```python
from build123d import *

# Parameters (mm, degrees)
F0_R     = 2
F0_R_2   = 4.5
F0_R_3   = 5.5
F1_DEPTH = 10
F0_R_4   = 3
F2_DEPTH = 4
F3_R     = 4
F3_R_2   = 2
F4_DEPTH = 5


with BuildPart() as f1:
    # F0 (on Front) → F1 (new body)
    with BuildSketch(Plane.XZ):
        with BuildLine():
            Line((20, -40), (10, 0))
            ThreePointArc((10, 0), (0, 10), (-10, 0))
            Line((-10, 0), (-20, -40))
            ThreePointArc((-20, -40), (0, -60), (20, -40))
        make_face()
        with Locations((-12.5, -40)):
            Circle(F0_R, mode=Mode.SUBTRACT)
        with Locations((0, -49.5)):
            Circle(F0_R, mode=Mode.SUBTRACT)
        with Locations((0, -40)):
            Circle(F0_R_2, mode=Mode.SUBTRACT)
        with Locations((0, -30.5)):
            Circle(F0_R, mode=Mode.SUBTRACT)
        with Locations((12.5, -40)):
            Circle(F0_R, mode=Mode.SUBTRACT)
        Circle(F0_R_3, mode=Mode.SUBTRACT)
    extrude(amount=F1_DEPTH)

    # F0 (on Front) → F2 (join)
    with BuildSketch(Plane.XZ):
        Circle(F0_R_3)
        Circle(F0_R_4, mode=Mode.SUBTRACT)
    extrude(amount=F2_DEPTH)

    # F3 (on face) → F4 (cut)
    with BuildSketch(Plane.XZ.offset(10)):
        with Locations((0, -30.5)):
            Circle(F3_R)
        with Locations((0, -30.5)):
            Circle(F3_R_2, mode=Mode.SUBTRACT)
        with Locations((-12.5, -40)):
            Circle(F3_R)
        with Locations((-12.5, -40)):
            Circle(F3_R_2, mode=Mode.SUBTRACT)
        with Locations((0, -49.5)):
            Circle(F3_R)
        with Locations((0, -49.5)):
            Circle(F3_R_2, mode=Mode.SUBTRACT)
        with Locations((12.5, -40)):
            Circle(F3_R)
        with Locations((12.5, -40)):
            Circle(F3_R_2, mode=Mode.SUBTRACT)
    extrude(amount=-F4_DEPTH, mode=Mode.SUBTRACT)


solid = f1.part
```
Could you check a few things on this model? Use its own coordinates, in mm. A direction names the side the tool comes from. Round coordinates to 2 decimals unless told otherwise and drop trailing zeros. Loops run counter-clockwise (first coordinate to the right, second up) from the corner with the lowest first, then second, coordinate; pieces in that order, holes last. Notation, with made-up numbers: (63.5, 35) -> (111.5, 35) arc R33 cw to (111.5, 67) -> close; hole circle Ø3 at (47.5, 25). An arc over 180 degrees is marked (long way). Put each result on its own line as item: value.
Q1. For pin 1 Ø5 at (x, y) = (14, -9) entering from -Z; pin 2 Ø3 at (x, y) = (-13.5, -1.5) entering from -Z; pin 3 Ø6 at (x, y) = (-6, -8) entering from -Z, each with a flat end and sliding along its axis, tell me the tip position at first contact or that it passes through.
Checks:
pin 1: z = -56.36
pin 2: z = -56
pin 3: z = -59.77
Q2. I want a section at A-A on x = 0. Give the number of separate pieces and of enclosed holes in the cut face, and give its area (3 significant figures).
Checks:
separate pieces: 5
enclosed holes: 0
area: 400 mm2
Q3. Please list where these lines run through material, in increasing order: line 1 (Z direction, x = 0, y = -6.9); line 2 (Z direction, x = 0, y = -2.7); line 3 (X direction, y = -0.75, z = -26). Write a range as from..to.
Checks:
line 1: -60..-53.5, -45.5..-44.5, -35.5..-34.5, -26.5..-5.5, 5.5..10
line 2: -60..-51.5, -47.5..-44.5, -35.5..-32.5, -28.5..-3, 3..10
line 3: -16.5..16.5
Q4. Which directions (+Z, -Z, +X, -X, +Y, -Y) give clear straight access to the entire face, cutting with the end or side of a thin tool? Please do faces 1 (the flat face through (2.4, -4, -2.4)), 2 (the cylindrical face through (0.923, -2.465, -51.274)).
Checks:
face 1: -Y
face 2: +Y, -Y
Q5. I want a section at D-D on z = -30.5. Write out the boundary of the cut face in (x, y) (3 decimals).
Checks:
outline: (-17.625, -10) -> (-4, -10) -> (-4, -5) -> (-2, -5) -> (-2, 0) -> (-17.625, 0) -> close; (2, -5) -> (4, -5) -> (4, -10) -> (17.625, -10) -> (17.625, 0) -> (2, 0) -> close
Q6. Thinking about a two-plate mould opening in Z: for faces 3 (the cylindrical face through (-0.98, -4.93, -44.39)), 4 (the cylindrical face through (0, -5, 10)), 5 (the cylindrical face through (0, -5, -60)), which applies, pulls with the +Z half, pulls with the -Z half, needs draft (parallel to the pull), parting line crosses it, or undercut?
Checks:
face 3: undercut
face 4: pulls with the +Z half
face 5: pulls with the -Z half
Q7. I want a section at C-C on x = 12.5. Write out the boundary of the cut face in (y, z), and give its area (3 significant figures).
Checks:
outline: (-10, -55.61) -> (0, -55.61) -> (0, -42) -> (-5, -42) -> (-5, -44) -> (-10, -44) -> close; (-10, -36) -> (-5, -36) -> (-5, -38) -> (0, -38) -> (0, -10) -> (-10, -10) -> close
area: 396 mm2
Q8. I want a section at B-B on y = -9. Write out the boundary of the cut face in (x, z), and give its area (3 significant figures).
Checks:
outline: (-20, -40) arc R20 ccw to (20, -40) -> (10, 0) arc R10 ccw to (-10, 0) -> close; hole circle Ø8 at (-12.5, -40); hole circle Ø11 at (0, 0); hole circle Ø9 at (0, -40); hole circle Ø8 at (0, -49.5); hole circle Ø8 at (0, -30.5); hole circle Ø8 at (12.5, -40)
area: 1,630 mm2
